The listing builds one solid part. Answer for the finished solid, in the listing's coordinates (mm). Coordinates: 2 decimals unless noted, no trailing zeros. Loops run counter-clockwise (first coordinate to the right, second up) from the corner with the lowest first, then second, coordinate; pieces in that order, holes last. Notation, with made-up numbers: M -4,-3.5 L 14,-3.5 A33 ccw 14,24.5 Z; hole C 70,7 d4. An arc over 180 degrees is marked long. Return JSON: item names as keys, results as strings. Group by question number.
1. Straight lines are drawn through the part: L1, parallel to X at y = 17, z = 0.95; L2, parallel to Y at x = 210, z = 1.2; L3, parallel to X at y = 15.5, z = 0.25. For each, find the intervals that lie inside material, in ascending order. Write a range as from..to.
2. Section B-B (x = 17.5) is taken. Write down the section's boundary in (y, z).
3. The mould has two halves that part along Y. Classify faces 1 (the face through (148, 18, 0)), 2 (the face through (15, 17.6, 1)), 3 (the face through (1, 2, 1)): pulls with the +Y half, pulls with the -Y half, needs draft (parallel to the pull), parting line crosses it, or undercut.
4. Section C-C (z = 1) is taken. Write down the section's boundary in (x, y).
5. Section A-A (y = 17.5) is taken. Write down the section's boundary in (x, z).
```python
from build123d import *

# Parameters (mm, degrees)
F0_W     = 300
F0_H     = 35
F0_R     = 2.5
F1_DEPTH = 2
F2_R     = 5
F3_SIZE2 = 41.2121612918
F3_SIZE  = 15


with BuildPart() as f1:
    # F0 (on Top) → F1 (new body)
    with BuildSketch(Plane.XY):
        with Locations((150, 17.5)):
            Rectangle(F0_W, F0_H)
        with Locations((17.5, 17.5)):
            Circle(F0_R, mode=Mode.SUBTRACT)
        with Locations((210, 17.5)):
            Circle(F0_R, mode=Mode.SUBTRACT)
    extrude(amount=F1_DEPTH)

    # F2
    f2_edges = [f1.edges().sort_by_distance(p)[0] for p in [
        (0, 0, 1),
        (300, 35, 1),
    ]]
    fillet(f2_edges, radius=F2_R)

    # F3
    f3_edges = [f1.edges().sort_by_distance(p)[0] for p in [
        (300, 0, 1),
    ]]
    f3_side = f1.faces().sort_by_distance((300, 15, 1))[0]
    chamfer(f3_edges, length=F3_SIZE, length2=F3_SIZE2, reference=f3_side)


solid = f1.part
```
Worked out:
{
 "1": {"L1": "0..15.05, 19.95..207.55, 212.45..300", "L2": "0..15, 20..35", "L3": "0..16, 19..208.5, 211.5..300"},
 "2": {"outline": "M 0,0 L 15,0 L 15,2 L 0,2 Z; M 20,0 L 35,0 L 35,2 L 20,2 Z"},
 "3": {"face 1": "needs draft", "face 2": "undercut", "face 3": "pulls with the -Y half"},
 "4": {"outline": "M 0,5 A5 ccw 5,0 L 258.79,0 L 300,15 L 300,30 A5 ccw 295,35 L 0,35 Z; hole C 17.5,17.5 d5; hole C 210,17.5 d5"},
 "5": {"outline": "M 0,0 L 15,0 L 15,2 L 0,2 Z; M 20,0 L 207.5,0 L 207.5,2 L 20,2 Z; M 212.5,0 L 300,0 L 300,2 L 212.5,2 Z"}
}
